Check sheet for the modelled part. Datum: model origin and axes. Units: mm. Face numbers are marked on the shaded views. A direction names the side the tool comes from. Coordinates: 2 decimals unless noted, no trailing zeros. Loops run counter-clockwise (first coordinate to the right, second up) from the corner with the lowest first, then second, coordinate; pieces in that order, holes last. Notation, with made-up numbers: M 8.5,38 L 29.5,38 A34 ccw 29.5,75 Z; hole C -27.75,51 d9. An arc over 180 degrees is marked long. Use CSV: the item, a comma, the result in double quotes. Start each with the question number.
(1) Section check D-D on x = -104.5. Record the cut outline in (y, z).
(2) Scan lines: line 1 (X direction, y = 57, z = -10.75); line 2 (Y direction, x = -106.75, z = -12); line 3 (Y direction, x = -96, z = -7). Record each from-to range of solid material in increasing order.
(3) Set-up check for the marked faces 5, 6 and 7: record each of +Z, -Z, +X, -X, +Y, -Y from which the full face is reachable in a straight line by a thin tool's end or side.
(4) Section check B-B on z = -8.5. Record the cut outline in (x, y), and give its area (3 significant figures).
(5) Draft check along Y on the marked faces 1, 2, 3 and 4. Enter one of: pulls with the +Y half, pulls with the -Y half, needs draft (parallel to the pull), parting line crosses it, or undercut.
(6) Section check A-A on y = 6.35. Record the cut outline in (x, z), and give its area (3 significant figures).
(7) Section check C-C on x = -96.25. Record the cut outline in (y, z), and give its area (3 significant figures).
(8) Go/stop test with flat-tipped pins: pin 1 Ø1.9 at (y, z) = (39.5, -8) entering from +X; pin 2 Ø5.5 at (x, y) = (-95.25, 57.15) entering from -Z. Record where each tip stops, or that it passes through.
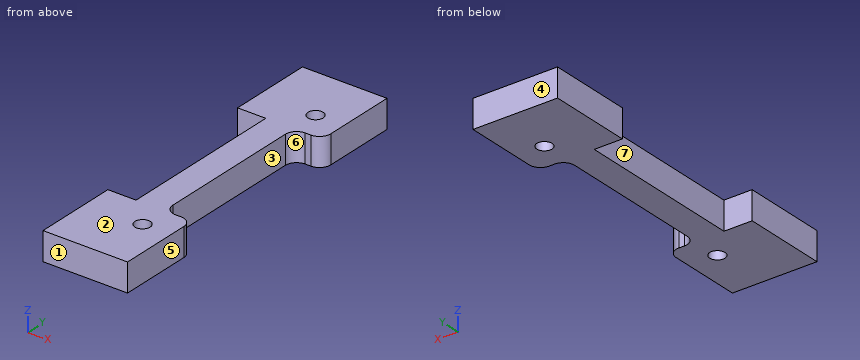
from build123d import *

# Parameters (mm, degrees)
BOSS_EXTRUDE1_START = -6.35
BOSS_EXTRUDE1_DEPTH = 6.35
FILLET1_R           = 2.54
SKETCH2_R           = 1.7272
CUT_EXTRUDE1_DEPTH  = 129.734406823


with BuildPart() as part:
    # Sketch1 → Boss-Extrude1 (new body)
    with BuildSketch(Plane.XY.offset(BOSS_EXTRUDE1_START)):
        Polygon((-107.95, -6.35), (-88.9, -6.35), (-88.9, 12.7), (-95.25, 12.7), (-95.25, 50.8), (-88.9, 50.8), (-88.9, 69.85), (-107.95, 69.85), (-107.95, 50.8), (-101.6, 50.8), (-101.6, 12.7), (-107.95, 12.7), align=None)
    extrude(amount=-BOSS_EXTRUDE1_DEPTH)

    # Fillet1
    fillet1_edges = [part.edges().sort_by_distance(p)[0] for p in [
        (-88.9, 50.8, -9.525),
        (-95.25, 50.8, -9.525),
        (-95.25, 12.7, -9.525),
        (-88.9, 12.7, -9.525),
    ]]
    fillet(fillet1_edges, radius=FILLET1_R)

    # Sketch2 → Cut-Extrude1 (cut, through all)
    with BuildSketch(Plane.XY.offset(-6.35)):
        with Locations((-95.25, 6.35)):
            Circle(SKETCH2_R)
        with Locations((-95.25, 57.15)):
            Circle(SKETCH2_R)
    extrude(amount=-CUT_EXTRUDE1_DEPTH, mode=Mode.SUBTRACT)


solid = part.part
Outcome:
1,outline,"M -6.35,-12.7 L 12.7,-12.7 L 12.7,-6.35 L -6.35,-6.35 Z; M 50.8,-12.7 L 69.85,-12.7 L 69.85,-6.35 L 50.8,-6.35 Z"
2,line 1,"x = -107.95 to -96.97, -93.53 to -88.9"
2,line 2,"y = -6.35 to 12.7, 50.8 to 69.85"
2,line 3,"y = -6.35 to 4.79, 7.91 to 55.59, 58.71 to 69.85"
3,face 5,"+Z, -Z, +X, +Y, -Y"
3,face 6,"+Z, -Z, +X"
3,face 7,"+Z, -Z, -X"
4,outline,"M -107.95,-6.35 L -88.9,-6.35 L -88.9,10.16 A2.54 ccw -91.44,12.7 L -92.71,12.7 A2.54 cw -95.25,15.24 L -95.25,48.26 A2.54 cw -92.71,50.8 L -91.44,50.8 A2.54 ccw -88.9,53.34 L -88.9,69.85 L -107.95,69.85 L -107.95,50.8 L -101.6,50.8 L -101.6,12.7 L -107.95,12.7 Z; hole C -95.25,6.35 d3.45; hole C -95.25,57.15 d3.45"
4,area,"949 mm²"
5,face 1,"pulls with the -Y half"
5,face 2,"needs draft"
5,face 3,"undercut"
5,face 4,"pulls with the +Y half"
6,outline,"M -107.95,-12.7 L -96.98,-12.7 L -96.98,-6.35 L -107.95,-6.35 Z; M -93.52,-12.7 L -88.9,-12.7 L -88.9,-6.35 L -93.52,-6.35 Z"
6,area,"99.0 mm²"
7,outline,"M -6.35,-12.7 L 4.94,-12.7 L 4.94,-6.35 L -6.35,-6.35 Z; M 7.76,-12.7 L 55.74,-12.7 L 55.74,-6.35 L 7.76,-6.35 Z; M 58.56,-12.7 L 69.85,-12.7 L 69.85,-6.35 L 58.56,-6.35 Z"
7,area,"448 mm²"
8,pin 1,"stops at x = -95.25"
8,pin 2,"stops at z = -12.7"
